```python
from build123d import *

# Parameters (mm, degrees)
EXTRUDE_1_DEPTH     = 3
SKETCH_2_R          = 1.5
CUT_EXTRUDE_1_DEPTH = 15.357381377


with BuildPart() as part:
    # 草图1 → 凸台-拉伸1 (new body)
    with BuildSketch(Plane.XY):
        with BuildLine():
            ThreePointArc((-4, 5.12), (0, 3.12), (4, 5.12))
            Line((4, 5.12), (4, 8.12))
            Line((4, 8.12), (-4, 8.12))
            Line((-4, 8.12), (-4, 5.12))
        make_face()
        with BuildLine():
            Line((4, 8.12), (4, 5.12))
            ThreePointArc((4, 5.12), (4.74341649, 6.53886117), (5, 8.12))
            ThreePointArc((5, 8.12), (-1.58113883, 12.86341649), (-4, 5.12))
            Line((-4, 5.12), (-4, 8.12))
            Line((-4, 8.12), (4, 8.12))
        make_face()
        with BuildLine():
            ThreePointArc((-4, -5.12), (0, -3.12), (4, -5.12))
            Line((4, -5.12), (4, 5.12))
            ThreePointArc((4, 5.12), (0, 3.12), (-4, 5.12))
            Line((-4, 5.12), (-4, -5.12))
        make_face()
        with BuildLine():
            Line((4, -5.12), (4, -8.12))
            Line((4, -8.12), (-4, -8.12))
            Line((-4, -8.12), (-4, -5.12))
            ThreePointArc((-4, -5.12), (-1.58113883, -12.86341649), (5, -8.12))
            ThreePointArc((5, -8.12), (4.74341649, -6.53886117), (4, -5.12))
        make_face()
        with BuildLine():
            Line((-4, -8.12), (4, -8.12))
            Line((4, -8.12), (4, -5.12))
            ThreePointArc((4, -5.12), (0, -3.12), (-4, -5.12))
            Line((-4, -5.12), (-4, -8.12))
        make_face()
    extrude(amount=EXTRUDE_1_DEPTH)

    # 草图2 → 切除-拉伸1 (cut, through all)
    with BuildSketch(Plane(origin=(0, 0, 0), x_dir=(-1, 0, 0), z_dir=(0, 0, -1))):
        with Locations((0, 8.12)):
            Circle(SKETCH_2_R)
        with Locations(Location((0, -8.12, 0), (0, 0, 180))):
            Circle(SKETCH_2_R)
    extrude(amount=-CUT_EXTRUDE_1_DEPTH, mode=Mode.SUBTRACT)


solid = part.part
```
Input: part model. Units: mm. Frame: model coordinates. Coordinates: 2 decimals unless noted, no trailing zeros. Loops run counter-clockwise (first coordinate to the right, second up) from the corner with the lowest first, then second, coordinate; pieces in that order, holes last. Notation, with made-up numbers: M 15,83.25 L 54,83.25 A6 cw 54,91.25 Z; hole C 20,11.5 d9. An arc over 180 degrees is marked long. Use a Markdown table: item, result. Add a question column.
1) Section A-A, the plane z = 2.4. Return the cut outline in (x, y), plus the area to 3 significant figures.
2) Section D-D, the plane x = -1. Return the cut outline in (y, z), plus the area to 3 significant figures.
3) Section C-C, the plane y = 0.5. Return the cut outline in (x, z).
4) Pin query (flat end, axial travel): P1, Ø1, axis at x = 2, z = 1.5, coming from the +Y side; P2, Ø1, axis at y = -3, z = 1.5, coming from the -X side; P3, Ø4, axis at x = 0, y = 8.12, coming from the -Z side. Return the tip coordinate at first contact, or that it passes through.
5) Draft query along Y for faces 1 (the flat face through (-4, 0, 1)), 2 (the flat face through (0, 0, 3)), 3 (the flat face through (4, 0, 1)). Return one class per face: +Y half, -Y half, draft (parallel to the pull), parting line (faces both ways), or undercut.
6) Section B-B, the plane x = 0. Return the cut outline in (y, z), plus the area to 3 significant figures.
7) Line query: L1, parallel to Y at x = 0, z = 2.3; L2, parallel to X at y = 8, z = 1.05; L3, parallel to Y at x = -0.5, z = 1.5. Output: solid intervals per line, ascending. Write a range as from..to.
Answer below:
| question | item | result |
|---|---|---|
| 1 | outline | M -4,-5.12 A5 ccw long 4,-5.12 L 4,5.12 A5 ccw long -4,5.12 Z; hole C 0,-8.12 d3; hole C 0,8.12 d3 |
| 1 | area | 202 mm2 |
| 2 | outline | M -13.02,0 L -9.24,0 L -9.24,3 L -13.02,3 Z; M -7,0 L 7,0 L 7,3 L -7,3 Z; M 9.24,0 L 13.02,0 L 13.02,3 L 9.24,3 Z |
| 2 | area | 64.7 mm2 |
| 3 | outline | M -4,0 L 4,0 L 4,3 L -4,3 Z |
| 4 | P1 | y = 12.89 |
| 4 | P2 | x = -4 |
| 4 | P3 | z = 0 |
| 5 | face 1 | undercut |
| 5 | face 2 | draft |
| 5 | face 3 | undercut |
| 6 | outline | M -13.12,0 L -9.62,0 L -9.62,3 L -13.12,3 Z; M -6.62,0 L 6.62,0 L 6.62,3 L -6.62,3 Z; M 9.62,0 L 13.12,0 L 13.12,3 L 9.62,3 Z |
| 6 | area | 60.7 mm2 |
| 7 | L1 | -13.12..-9.62, -6.62..6.62, 9.62..13.12 |
| 7 | L2 | -5..-1.5, 1.5..5 |
| 7 | L3 | -13.09..-9.53, -6.71..6.71, 9.53..13.09 |
